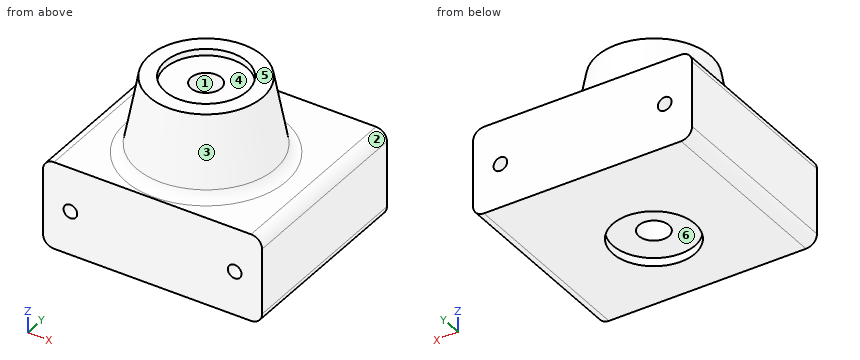
from build123d import *

# Parameters (mm, degrees)
SKETCH_1_W             = 40
SKETCH_1_H             = 35
EXTRUDE_457_DEPTH      = 16
SKETCH_2_R             = 10
EXTRUDE_593_DEPTH      = 14
SKETCH_4_R             = 2.75
CUT_EXTRUDE_684_DEPTH  = 42.231056256
CHAMFER_2_SIZE         = 3
CHAMFER_2_SIZE_2       = 16
FILLET_5_R             = 2
SKETCH_7_R             = 1.25
CUT_EXTRUDE_1001_DEPTH = 44.370496884
FILLET_7_R             = 2
SKETCH_8_R             = 7.5
CUT_EXTRUDE_1355_DEPTH = 1.2
CUT_EXTRUDE_START      = -1.5
SKETCH_9_R             = 7.5
CUT_EXTRUDE_1489_DEPTH = 1.5


with BuildPart() as part:
    # Эскиз1 → Extrude 457 (new body)
    with BuildSketch(Plane.XY):
        with Locations((0, 2.5)):
            Rectangle(SKETCH_1_W, SKETCH_1_H)
    extrude(amount=-EXTRUDE_457_DEPTH)

    # Эскиз2 → Extrude 593 (add)
    with BuildSketch(Plane.XY):
        Circle(SKETCH_2_R)
    extrude(amount=EXTRUDE_593_DEPTH)

    # Эскиз4 → Cut-Extrude 684 (cut, through all)
    with BuildSketch(Plane.XY.offset(14)):
        Circle(SKETCH_4_R)
    extrude(amount=-CUT_EXTRUDE_684_DEPTH, mode=Mode.SUBTRACT)

    # Фаска2
    # the kernel refuses this chamfer: 16, 3 mm, written as the material it adds along each edge
    with BuildSketch(Plane(origin=(0, 0, 0), x_dir=(1, 0, 0), z_dir=(0, -1, 0))) as chamfer_2_piece_1_section:
        Polygon((10 + CHAMFER_2_SIZE, 0), (10, CHAMFER_2_SIZE_2), (10, 0), align=None)
    chamfer_2_piece_1 = revolve(axis=Axis((0, 0, 0), (0, 0, 1)), mode=Mode.PRIVATE)
    chamfer_2_piece_1 = split(chamfer_2_piece_1, bisect_by=Plane(origin=(-11.622307858, 0, 14), z_dir=(0, 0, -1)), keep=Keep.TOP, mode=Mode.PRIVATE)
    add(chamfer_2_piece_1)

    # Скругление5
    fillet_5_edges = [part.edges().sort_by_distance(p)[0] for p in [
        (-13, 0, 0),
    ]]
    fillet(fillet_5_edges, radius=FILLET_5_R)

    # Эскиз7 → Cut-Extrude 1001 (cut, through all)
    with BuildSketch(Plane(origin=(0, 20, 0), x_dir=(1, 0, 0), z_dir=(0, 1, 0))):
        with Locations(Location((-15, 8, 0), (0, 0, 180))):
            Circle(SKETCH_7_R)
        with Locations(Location((15, 8, 0), (0, 0, 180))):
            Circle(SKETCH_7_R)
    extrude(amount=-CUT_EXTRUDE_1001_DEPTH, mode=Mode.SUBTRACT)

    # Скругление7
    fillet_7_edges = [part.edges().sort_by_distance(p)[0] for p in [
        (20, 2.5, -16),
        (-20, 2.5, -16),
        (20, 2.5, 0),
        (-20, 2.5, 0),
    ]]
    fillet(fillet_7_edges, radius=FILLET_7_R)

    # Эскиз8 → Cut-Extrude 1355 (cut)
    with BuildSketch(Plane.XY.offset(14)):
        Circle(SKETCH_8_R)
    extrude(amount=-CUT_EXTRUDE_1355_DEPTH, mode=Mode.SUBTRACT)

    # Эскиз9 → Cut-Extrude 1489 (cut)
    with BuildSketch(Plane(origin=(0, 0, -16), x_dir=(-1, 0, 0), z_dir=(0, 0, -1)).offset(CUT_EXTRUDE_START)):
        with Locations(Location((0, 0, 0), (0, 0, 180))):
            Circle(SKETCH_9_R)
    extrude(amount=CUT_EXTRUDE_1489_DEPTH, mode=Mode.SUBTRACT)


solid = part.part
Here's how the part is built. I have some questions about the finished solid (model axes, mm). Face numbers are marked on the shaded views. A direction names the side the tool comes from. Give positions to 0.01 mm unless a question says otherwise; leave off trailing zeros. Loops run counter-clockwise (first coordinate to the right, second up) from the corner with the lowest first, then second, coordinate; pieces in that order, holes last. Notation, with made-up numbers: (79.25, 70) -> (131.25, 70) arc R9 ccw to (131.25, 84) -> close; hole circle Ø5 at (-36, 55.25). An arc over 180 degrees is marked (long way). Answer as a JSON object with one key per item and string values. Group by question number.
Item 1: Imagine slicing it at B-B on y = 17. Write out the boundary of the cut face in (x, z), then the cut area to 3 significant figures.
Item 2: On a 3-axis mill with a long thin cutter (end or side, diameter ignored), from which of +Z, -Z, +X, -X, +Y, -Y can I reach the whole of each face in a straight line? I mean the marked faces 4, 5 and 6. Say none if no direction works.
Item 3: Thinking about a two-plate mould opening in Y: for the marked faces 1, 2 and 3, which applies, pulls with the +Y half, pulls with the -Y half, needs draft (parallel to the pull), parting line crosses it, or undercut?
Item 4: Will these pins go through, and if not, where does the flat tip stop? pin 1 (10 mm diameter, centred on y = 5.5, z = 10.5, fed in from +X); pin 2 (4.5 mm diameter, centred on x = 3.5, y = 3.5, fed in from -Z); pin 3 (6 mm diameter, centred on x = -11.5, z = 6.5, fed in from -Y).
Item 5: Imagine slicing it at C-C on x = 0. Write out the boundary of the cut face in (y, z) (3 decimals).
Item 6: Imagine slicing it at A-A on y = 0. Write out the boundary of the cut face in (x, z) (3 decimals).
Item 7: Imagine slicing it at D-D on z = -6. Write out the boundary of the cut face in (x, y).
Item 8: I need wall thicknesses on L1, parallel to Z at x = 15, y = 9.5; L2, parallel to Z at x = 18, y = 14; L3, parallel to Y at x = 0, z = 0.5. Which ranges of each line are inside material? Lowest first, please.
Answer list:
{
 "1": {"outline": "(-20, -14) arc R2 ccw to (-18, -16) -> (18, -16) arc R2 ccw to (20, -14) -> (20, -2) arc R2 ccw to (18, 0) -> (-18, 0) arc R2 ccw to (-20, -2) -> close; hole circle Ø2.5 at (-15, -8); hole circle Ø2.5 at (15, -8)", "area": "627 mm2"},
 "2": {"face 4": "+Z", "face 5": "+Z, +X, -X, +Y, -Y", "face 6": "-Z"},
 "3": {"face 1": "undercut", "face 2": "needs draft", "face 3": "parting line crosses it"},
 "4": {"pin 1": "stops at x = 11.53", "pin 2": "stops at z = -14.5", "pin 3": "stops at y = -8.26"},
 "5": {"outline": "(-15, -16) -> (-7.5, -16) -> (-7.5, -14.5) -> (-2.75, -14.5) -> (-2.75, 12.8) -> (-7.5, 12.8) -> (-7.5, 14) -> (-10.375, 14) -> (-12.694, 1.631) arc R2 cw to (-14.66, 0) -> (-15, 0) -> close; (2.75, -14.5) -> (7.5, -14.5) -> (7.5, -16) -> (20, -16) -> (20, 0) -> (14.66, 0) arc R2 cw to (12.694, 1.631) -> (10.375, 14) -> (7.5, 14) -> (7.5, 12.8) -> (2.75, 12.8) -> close"},
 "6": {"outline": "(-20, -14) arc R2 ccw to (-18, -16) -> (-7.5, -16) -> (-7.5, -14.5) -> (-2.75, -14.5) -> (-2.75, 12.8) -> (-7.5, 12.8) -> (-7.5, 14) -> (-10.375, 14) -> (-12.694, 1.631) arc R2 cw to (-14.66, 0) -> (-18, 0) arc R2 ccw to (-20, -2) -> close; (2.75, -14.5) -> (7.5, -14.5) -> (7.5, -16) -> (18, -16) arc R2 ccw to (20, -14) -> (20, -2) arc R2 ccw to (18, 0) -> (14.66, 0) arc R2 cw to (12.694, 1.631) -> (10.375, 14) -> (7.5, 14) -> (7.5, 12.8) -> (2.75, 12.8) -> close; hole circle Ø2.5 at (-15, -8); hole circle Ø2.5 at (15, -8)"},
 "7": {"outline": "(-20, -15) -> (20, -15) -> (20, 20) -> (-20, 20) -> close; hole circle Ø5.5 at (0, 0)"},
 "8": {"L1": "z = -16 to -9.25, -6.75 to 0", "L2": "z = -16 to 0", "L3": "y = -13.34 to -2.75, 2.75 to 13.34"}
}
